Autodesk Inventor part; units mm, degrees
ref_plane "YZ Plane" through (0, 0, 0) normal (1, 0, 0) x (0, 1, 0)
ref_plane "XZ Plane" through (0, 0, 0) normal (0, 1, 0) x (-1, 0, 0)
ref_plane "XY Plane" through (0, 0, 0) normal (0, 0, 1) x (1, 0, 0)
sketch "Sketch1" plane through (0, 0, 0) normal (0, 0, 1) x (1, 0, 0)
  circle A0 centre (0, 0) radius 1.5875
  circle A1 centre (0, 0) radius 3.175
  line L0 (0, 0) -> (36.2951, -20.955)
  line L1 (0, 0) -> (41.91, 0) construction
  circle A2 centre (36.2951, -20.955) radius 1.5875
  circle A3 centre (36.2951, -20.955) radius 3.175
  line L2 (0, 0) -> (0, 8.5417)
  circle A4 centre (-36.2951, -20.955) radius 1.5875
  circle A5 centre (-36.2951, -20.955) radius 3.175
  line L3 (-29.1831, -8.3058) -> (24.9189, -8.3058)
  line L4 (24.9189, -8.3058) -> (24.9189, -6.2738)
  line L5 (24.9189, -6.2738) -> (-29.1831, -6.2738)
  line L6 (-29.1831, -6.2738) -> (-29.1831, -8.3058)
  line L7 (-16.4831, -6.2738) -> (-16.4831, -8.3058)
  line L8 (-30.4531, -5.0038) -> (27.2049, -5.0038)
  line L9 (27.2049, -5.0038) -> (27.2049, -10.5918)
  line L10 (27.2049, -10.5918) -> (-30.4531, -10.5918)
  line L11 (-30.4531, -10.5918) -> (-30.4531, -5.0038)
  line L12 (-30.4531, -5.0038) -> (-0.8344, 3.0634)
  line L13 (-30.4531, -10.5918) -> (-38.5445, -18.7142)
  line L14 (27.2049, -5.0038) -> (0.6506, 3.1076)
  line L15 (27.2049, -10.5918) -> (38.1356, -18.3679)
  line L16 (34.4546, -23.5421) -> (16.2505, -10.5918)
  line L17 (-34.0458, -23.1958) -> (-21.49, -10.5918)
  dimension "d0" = 3.175
  dimension "d1" = 6.35
  dimension "d2" = 41.91
  dimension "d3" = 30
  dimension "d4" = 3.175
  dimension "d5" = 6.35
  dimension "d6" = 7.112
  dimension "d7" = 12.6492
  dimension "d8" = 54.102
  dimension "d9" = 41.402
  dimension "d10" = 1.27
  dimension "d11" = 2.286
  dimension "d12" = 1.27
  dimension "d13" = 2.286
  dimension "d16" = 2.032
extrude "Extrusion1" add sketch "Sketch1" along normal blind 2.8575 contours A0 L2 A1 L14 L0 | A0 L0 A1 L2 | L0 L8 L12 A1 | A1 L14 L8 L0 | L8 L9 L10 L0 L3 L4 L5 | L0 L5 L6 L3 L10 L11 L8 | L10 L17 A5 L13 | L15 A3 L0 L10 | A5 | L0 A3 L16 L10 | A3
fillet "Fillet1" radius 3.175 6 edges at (27.2049, -10.5918, 1.4287) (27.2049, -5.0038, 1.4287) (-30.4531, -5.0038, 1.4287) (-30.4531, -10.5918, 1.4287) (-21.49, -10.5918, 1.4287) (16.2505, -10.5918, 1.4287)
sketch "Sketch4" plane through (0, 0, 0) normal (0, 0, -1) x (-1, 0, 0)
  arc A0 (30.4531, -7.4297) -> (28.1125, -4.3663) centre (27.2781, -7.4297) ccw
  line L0 (0.8344, 3.0634) -> (28.1125, -4.3663)
  arc A1 (0.8344, 3.0634) -> (-0.6506, 3.1076) centre (0, 0) ccw
  line L1 (-24.9574, -4.3173) -> (-0.6506, 3.1076)
  arc A2 (-24.9574, -4.3173) -> (-27.2049, -7.3538) centre (-24.0299, -7.3538) ccw
  line L2 (-27.2049, -8.954) -> (-27.2049, -7.3538)
  arc A3 (-28.5394, -11.5412) -> (-27.2049, -8.954) centre (-30.3799, -8.954) ccw
  line L3 (-38.1356, -18.3679) -> (-28.5394, -11.5412)
  arc A4 (-38.1356, -18.3679) -> (-34.4546, -23.5421) centre (-36.2951, -20.955) ccw
  line L4 (-17.0769, -11.1797) -> (-34.4546, -23.5421)
  arc A5 (-15.2364, -10.5918) -> (-17.0769, -11.1797) centre (-15.2364, -13.7668) ccw
  line L5 (20.1713, -10.5918) -> (-15.2364, -10.5918)
  arc A6 (22.4207, -11.526) -> (20.1713, -10.5918) centre (20.1713, -13.7668) ccw
  line L6 (34.0458, -23.1958) -> (22.4207, -11.526)
  arc A7 (34.0458, -23.1958) -> (38.5445, -18.7142) centre (36.2951, -20.955) ccw
  line L7 (31.3788, -11.521) -> (38.5445, -18.7142)
  arc A8 (30.4531, -9.2802) -> (31.3788, -11.521) centre (33.6281, -9.2802) ccw
  line L8 (30.4531, -7.4297) -> (30.4531, -9.2802)
  circle A9 centre (36.2951, -20.955) radius 1.5875
  line L9 (29.1831, -8.3058) -> (-24.9189, -8.3058)
  line L10 (-24.9189, -8.3058) -> (-24.9189, -6.2738)
  line L11 (-24.9189, -6.2738) -> (29.1831, -6.2738)
  line L12 (29.1831, -6.2738) -> (29.1831, -8.3058)
  circle A10 centre (0, 0) radius 1.5875
  circle A11 centre (-36.2951, -20.955) radius 1.5875
  line L13 (-23.2186, 2.3851) -> (-3.81, 2.3851)
  line L14 (-3.81, 2.3851) -> (-3.81, -2.8268)
  line L15 (-3.81, -2.8268) -> (-23.2186, -2.8268)
  line L16 (-23.2186, -2.8268) -> (-23.2186, 2.3851)
  line L17 (23.7839, 2.3851) -> (3.81, 2.3851)
  line L18 (3.81, 2.3851) -> (3.81, -2.8268)
  line L19 (3.81, -2.8268) -> (23.7839, -2.8268)
  line L20 (23.7839, -2.8268) -> (23.7839, 2.3851)
  dimension "d23" = 3.81
  dimension "d24" = 3.81
extrude "Extrusion3" cut sketch "Sketch4" against normal through all contours L19 L18 L0 | L0 L18 L17 L20 L19 | L14 L15 L1 | L1 L15 L16 L13 L14
fillet "Fillet2" radius 3.175 6 edges at (3.81, 2.1425, 1.4287) (3.81, -2.8268, 1.4287) (-3.81, -2.8268, 1.4287) (-3.81, 2.2529, 1.4287) (20.0782, -2.8268, 1.4287) (-22.4604, -2.8268, 1.4287)
sketch "Sketch7" plane through (0, 0, 2.8575) normal (0, 0, 1) x (1, 0, 0)
  line L0 (-16.4831, -6.2738) -> (-16.4831, -8.3058)
  line L1 (-29.1831, -8.3058) -> (-29.1831, -6.2738)
  line L2 (-16.4831, -8.3058) -> (-29.1831, -8.3058)
  line L3 (-29.1831, -8.3058) -> (-29.1831, -6.2738)
  line L4 (-29.1831, -6.2738) -> (-16.4831, -6.2738)
  line L5 (-16.4831, -6.2738) -> (-16.4831, -8.3058)
  point P0 (0, 0)
extrude "Extrusion5" add sketch "Sketch7" against normal blind 0.508
properties part number "ArduinoMegaHolder1" material "ABS Plastic"
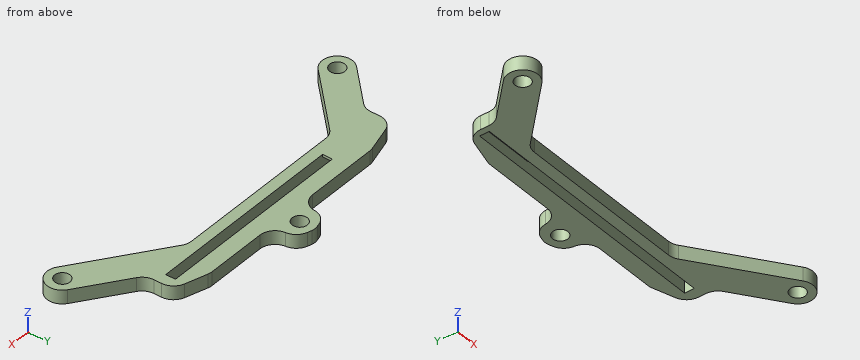
Design review of the part built by this model. Coordinates are the model's own, in mm. Coordinates: 2 decimals unless noted, no trailing zeros. Write each loop counter-clockwise with the first axis right and the second up, starting at its lowest first coordinate (ties: lowest second). Pieces come first, ordered by that corner, then holes. Notation, with made-up numbers: (56.5, -6.5) - (87.5, -6.5) arc R16 ccw to (87.5, 14.5) - close; hole circle Ø4 at (-6.75, 1). An arc over 180 degrees is marked (long way). One line per item, written item: value.
1) To check wall thickness, follow probe 1 along Y at (x, z) = (0, 2.05) (1 decimal); probe 2 along Y at (x, z) = (-20.5, 0.1); probe 3 along X at (y, z) = (-8.25, 1.75). State the ranges of each line that lie inside material, in increasing order.
Answer sheet:
probe 1: y = -10.6 to -8.3, -6.3 to -1.6, 1.6 to 3.2
probe 2: y = -10.61 to -8.31, -6.27 to -2.83
probe 3: x = -30.45 to -29.18, 24.92 to 27.2
2) Add section B-B (x = -32.5). State the section outline as (y, z) points, plus the area to 3 significant figures.
Answer sheet:
outline: (-21.64, 0) - (-12.65, 0) - (-12.65, 2.86) - (-21.64, 2.86) - close
area: 25.7 mm2
3) Add section A-A (z = 1.9). Give the number of separate pieces and of enclosed holes in the cut face, plus the area to 3 significant figures.
Answer sheet:
separate pieces: 1
enclosed holes: 4
area: 579 mm2
4) Insertion check: pin 1 (1.4 mm diameter, centred on x = -9, z = 1.5, fed in from -Y); pin 2 (0.6 mm diameter, centred on y = -7.5, z = 1, fed in from -X); pin 3 (2.5 mm diameter, centred on x = 36.3, y = -20.96, fed in from -Z); pin 4 (1 mm diameter, centred on x = -30, z = 1.5, fed in from +Y). Each pin has a flat end and moves straight along its axis. Give the tip position at first contact, or say it passes through.
Answer sheet:
pin 1: stops at y = -10.59
pin 2: stops at x = -30.45
pin 3: passes through
pin 4: stops at y = -5.16
